from build123d import *

# Parameters (mm, degrees)
F0_W     = 40
F0_H     = 40
F1_DEPTH = 17
F2_R     = 6
F3_DEPTH = 8.5
F4_R     = 7.5
F5_DEPTH = 3.5
F6_R     = 4
F7_W     = 24.5
F7_H     = 3
F8_DEPTH = 7


with BuildPart() as f1:
    # F0 (on Top) → F1 (new body)
    with BuildSketch(Plane.XY):
        Rectangle(F0_W, F0_H)
    extrude(amount=-F1_DEPTH)

    # F2 (on face) → F3 (join)
    with BuildSketch(Plane.XY):
        Circle(F2_R)
    extrude(amount=F3_DEPTH)

    # F4 (on face) → F5 (join)
    with BuildSketch(Plane.XY.offset(8.5)):
        Circle(F4_R)
    extrude(amount=F5_DEPTH)

    # F6
    f6_edges = [f1.edges().sort_by_distance(p)[0] for p in [
        (20, -20, -8.5),
        (20, 20, -8.5),
        (-20, 20, -8.5),
        (-20, -20, -8.5),
    ]]
    fillet(f6_edges, radius=F6_R)

    # F7 (on face) → F8 (cut)
    with BuildSketch(Plane.XZ.offset(20)):
        with Locations((0, -4.5)):
            Rectangle(F7_W, F7_H)
    extrude(amount=-F8_DEPTH, mode=Mode.SUBTRACT)


solid = f1.part
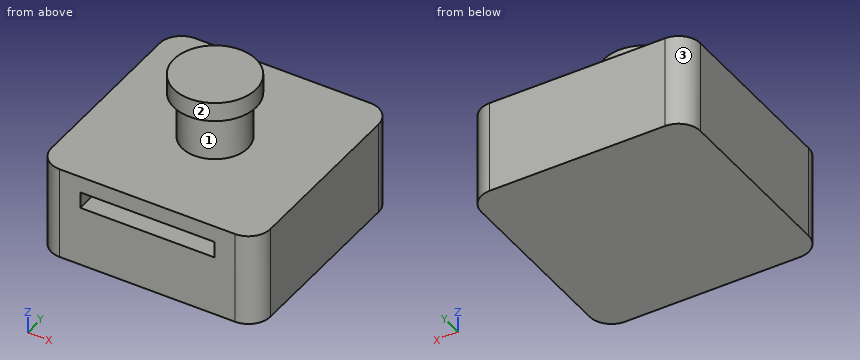
Geometry check sheet. Reference: the model listing, model coordinates, mm. Face numbers are marked on the shaded views. A direction names the side the tool comes from. Round coordinates to 2 decimals unless told otherwise and drop trailing zeros. Order: outer loops, then holes, each group sorted by start corner. A loop starts at its lowest first (then second) coordinate and runs counter-clockwise, first axis right, second up. Notation, with made-up numbers: M 18.25,-20 L 36.25,-20 A26 ccw 36.25,19 Z; hole C -9,-12 d4. An arc over 180 degrees is marked long. Answer in a Markdown table with one row per item. Add a question column.
Item 1: Sectioned sample at A-A, the plane y = 0. Enter the section's corners in (x, z), plus the area to 4 significant figures.
Item 2: Material ranges on L1, parallel to Z at x = 4, y = 5.5; L2, parallel to X at y = -16, z = -5.5; L3, parallel to Z at x = 6, y = 10, recorded low to high. Write a range as [from, to].
Item 3: Depth check by flat-ended pin: pin 1 Ø2 at (x, y) = (6, -15) entering from +Z; pin 2 Ø3 at (y, z) = (-9, 7.5) entering from +X; pin 3 Ø2.5 at (y, z) = (-18, -4) entering from -X; pin 4 Ø0.9 at (x, z) = (0, -4) entering from -Y. Enter the tip coordinate at first touch or a pass-through.
Item 4: Set-up check for the marked faces 1, 2 and 3: record each of +Z, -Z, +X, -X, +Y, -Y from which the full face is reachable in a straight line by a thin tool's end or side.
Item 5: Sectioned sample at C-C, the plane z = 4.25. Enter the section's corners in (x, y), plus the area to 3 significant figures.
Item 6: Sectioned sample at B-B, the plane x = 8.5. Enter the section's corners in (y, z), plus the area to 3 significant figures.
Item 7: Sectioned sample at D-D, the plane x = 0. Enter the section's corners in (y, z).
Filled in:
| question | item | result |
|---|---|---|
| 1 | outline | M -20,-17 L 20,-17 L 20,0 L 6,0 L 6,8.5 L 7.5,8.5 L 7.5,12 L -7.5,12 L -7.5,8.5 L -6,8.5 L -6,0 L -20,0 Z |
| 1 | area | 834.5 mm² |
| 2 | L1 | z = [-17, 0], [8.5, 12] |
| 2 | L2 | x = [-20, -12.25], [12.25, 20] |
| 2 | L3 | z = [-17, 0] |
| 3 | pin 1 | stops at z = 0 |
| 3 | pin 2 | passes through |
| 3 | pin 3 | stops at x = -19.93 |
| 3 | pin 4 | stops at y = -13 |
| 4 | face 1 | none |
| 4 | face 2 | +Z |
| 4 | face 3 | +Z, -Z, -X, +Y |
| 5 | outline | C 0,0 d12 |
| 5 | area | 113 mm² |
| 6 | outline | M -20,-17 L 20,-17 L 20,0 L -20,0 L -20,-3 L -13,-3 L -13,-6 L -20,-6 Z |
| 6 | area | 659 mm² |
| 7 | outline | M -20,-17 L 20,-17 L 20,0 L 6,0 L 6,8.5 L 7.5,8.5 L 7.5,12 L -7.5,12 L -7.5,8.5 L -6,8.5 L -6,0 L -20,0 L -20,-3 L -13,-3 L -13,-6 L -20,-6 Z |
